Could you check a few things on this drawing? It's one solid part, dimensions in mm from its lowest x, y, z. A direction names the side the tool comes from. Coordinates: 2 decimals unless noted, no trailing zeros. Write each loop counter-clockwise with the first axis right and the second up, starting at its lowest first coordinate (ties: lowest second). Pieces come first, ordered by that corner, then holes. Notation, with made-up numbers: M 23,-21 L 45,-21 A24 ccw 45,18 Z; hole C 17,-9.75 d4. An arc over 180 degrees is marked long. Use a Markdown table: item, result.
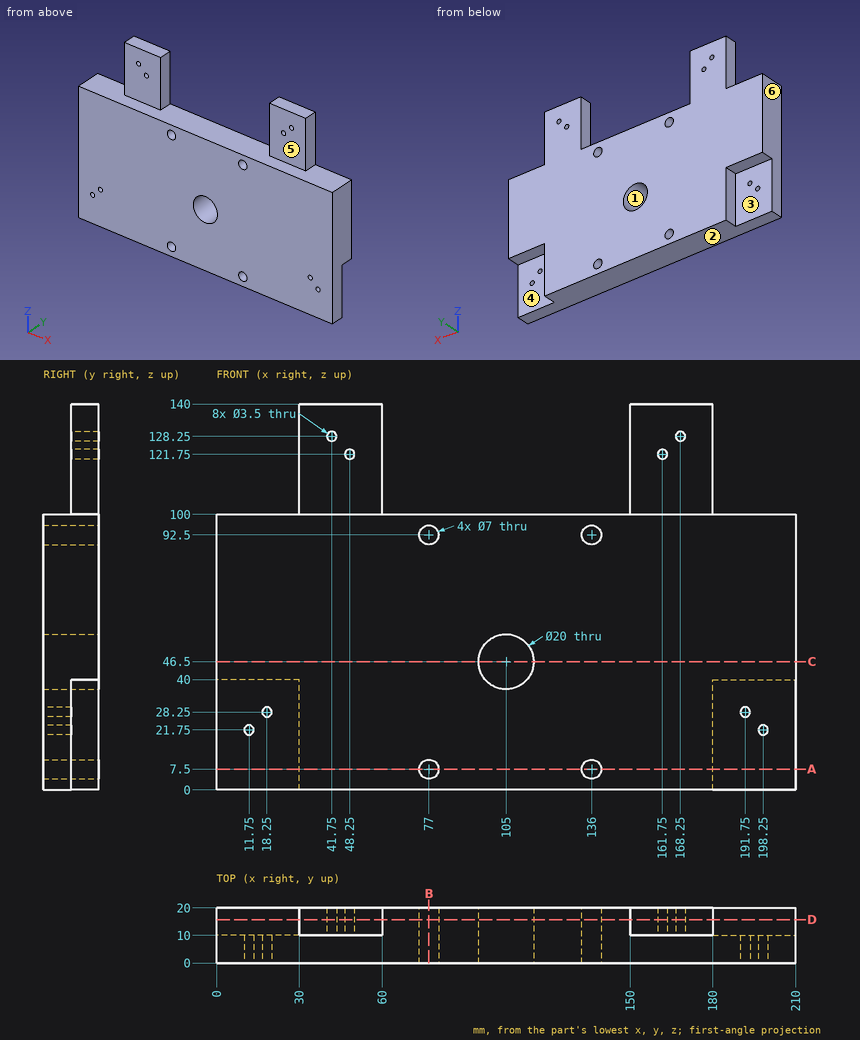
1. Which directions (+Z, -Z, +X, -X, +Y, -Y) give clear straight access to the entire face, cutting with the end or side of a thin tool? Please do the marked faces 4, 5 and 6.
Answers follow:
| item | result |
|---|---|
| face 4 | -Z, +X, +Y |
| face 5 | +Z, +X, -X, -Y |
| face 6 | +Z, -Z, -X, +Y, -Y |
2. We'd pull the mould along Z, two halves only. Please class the marked faces 1, 2 and 3: +Z half, -Z half, draft (parallel to the pull), parting line (faces both ways), or undercut.
Answers follow:
| item | result |
|---|---|
| face 1 | undercut |
| face 2 | -Z half |
| face 3 | draft |
3. Will these pins go through, and if not, where does the flat tip stop? pin 1 Ø3 at (x, z) = (198.25, 21.75) entering from -Y; pin 2 Ø3 at (x, y) = (76.5, 9) entering from +Z; pin 3 Ø1 at (x, y) = (24, 16) entering from -Z; pin 4 Ø24 at (x, z) = (165, 114.5) entering from -Y.
Answers follow:
| item | result |
|---|---|
| pin 1 | passes through |
| pin 2 | stops at z = 100 |
| pin 3 | stops at z = 40 |
| pin 4 | stops at y = 10 |
4. Suppose I cut it at A-A on z = 7.5. Write out the boundary of the cut face in (x, y).
Answers follow:
| item | result |
|---|---|
| outline | M 0,0 L 73.5,0 L 73.5,20 L 30,20 L 30,10 L 0,10 Z; M 80.5,0 L 132.5,0 L 132.5,20 L 80.5,20 Z; M 139.5,0 L 210,0 L 210,10 L 180,10 L 180,20 L 139.5,20 Z |
5. Suppose I cut it at C-C on z = 46.5. Write out the boundary of the cut face in (x, y).
Answers follow:
| item | result |
|---|---|
| outline | M 0,0 L 95,0 L 95,20 L 0,20 Z; M 115,0 L 210,0 L 210,20 L 115,20 Z |
6. Suppose I cut it at D-D on y = 15.75. State how many separate pieces and enclosed holes the cut face has, and give its area (3 significant figures).
Answers follow:
| item | result |
|---|---|
| separate pieces | 1 |
| enclosed holes | 9 |
| area | 20,500 mm2 |
7. Suppose I cut it at B-B on x = 77. Write out the boundary of the cut face in (y, z), and give its area (3 significant figures).
Answers follow:
| item | result |
|---|---|
| outline | M 0,0 L 20,0 L 20,4 L 0,4 Z; M 0,11 L 20,11 L 20,89 L 0,89 Z; M 0,96 L 20,96 L 20,100 L 0,100 Z |
| area | 1,720 mm2 |
8. I need wall thicknesses on probe 1 along X at (y, z) = (16.75, 121.75); probe 2 along X at (y, z) = (6.25, 28.25); probe 3 along X at (y, z) = (15.5, 128.25). Which ranges of each line are inside material? Lowest first, please.
Answers follow:
| item | result |
|---|---|
| probe 1 | x = 30 to 46.5, 50 to 60, 150 to 160, 163.5 to 180 |
| probe 2 | x = 0 to 16.5, 20 to 190, 193.5 to 210 |
| probe 3 | x = 30 to 40, 43.5 to 60, 150 to 166.5, 170 to 180 |
